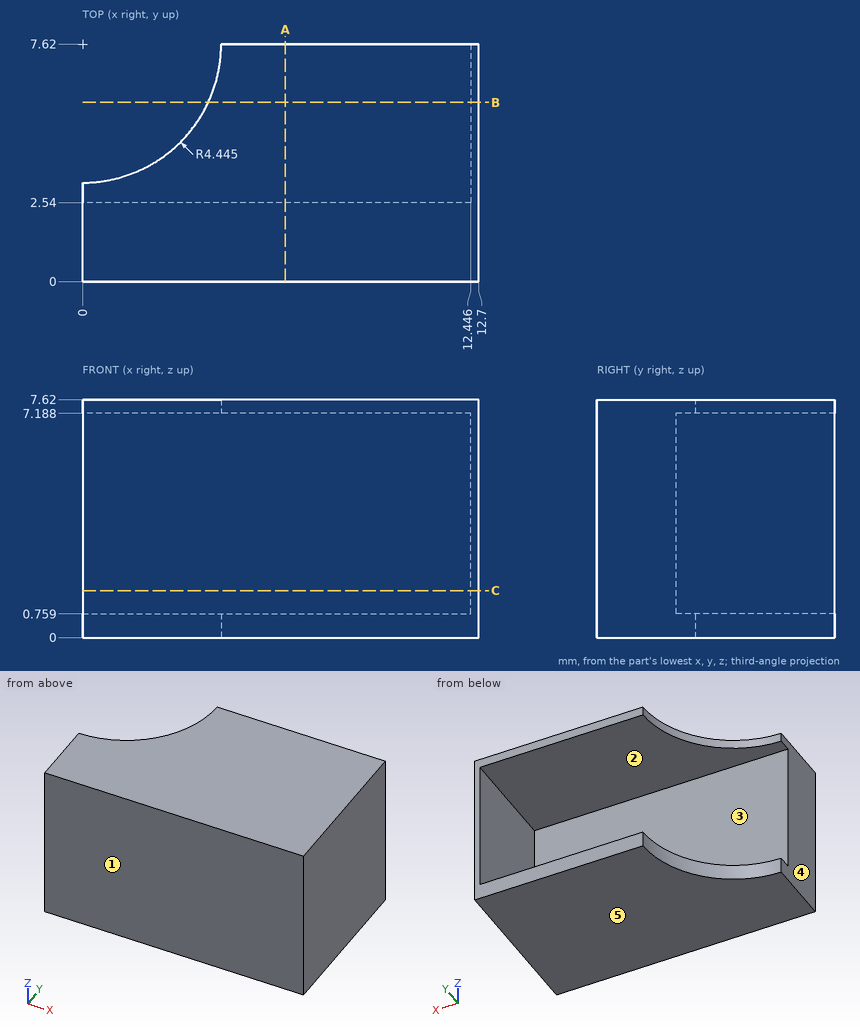
For this review, use the dimensioned drawing (mm, ordinates from the lowest corner) and the shaded views. A direction names the side the tool comes from. Coordinates: 2 decimals unless noted, no trailing zeros. Order: outer loops, then holes, each group sorted by start corner. A loop starts at its lowest first (then second) coordinate and runs counter-clockwise, first axis right, second up. Notation, with made-up numbers: (-26.5, 50.25) -> (3.5, 50.25) arc R19 cw to (3.5, 59.25) -> close; hole circle Ø4 at (-10, -35.75). An arc over 180 degrees is marked (long way). One line per item, written item: value. Start each with the question number.
Q1. Take a section at A-A, the plane x = 6.5. State the section outline as (y, z) points, then the cut area to 3 significant figures.
Q2. Take a section at C-C, the plane z = 1.5. State the section outline as (x, y) points.
Q3. For probe 1 along Z at (x, y) = (7, 4); probe 2 along X at (y, z) = (5, 2); probe 3 along Y at (x, z) = (11.25, 2.5), list the stretches that pass through material, from the lowest coordinate up.
Q4. Take a section at B-B, the plane y = 5.75. State the section outline as (x, z) points.
Q5. Insertion check: pin 1 Ø1.5 at (x, z) = (6, 3) entering from +Y. The pin has a flat end and moves straight along its axis. Give the tip position at first contact, or say it passes through.
Q6. Tool access review of the marked faces 1 and 2: name each direction out of +Z, -Z, +X, -X, +Y, -Y from which nothing blocks a thin tool from reaching the whole face with its end or side.
Q7. Mouldability with a two-part tool opening along Z and no side actions: class the marked faces 3, 4 and 5 as pulls with the +Z half, pulls with the -Z half, needs draft (parallel to the pull), parting line crosses it, or undercut.
Values follow:
1. outline: (0, 0) -> (7.62, 0) -> (7.62, 0.76) -> (2.54, 0.76) -> (2.54, 7.19) -> (7.62, 7.19) -> (7.62, 7.62) -> (0, 7.62) -> close
1. area: 25.4 mm2
2. outline: (0, 0) -> (12.7, 0) -> (12.7, 7.62) -> (12.45, 7.62) -> (12.45, 2.54) -> (0, 2.54) -> close
3. probe 1: z = 0 to 0.76, 7.19 to 7.62
3. probe 2: x = 12.45 to 12.7
3. probe 3: y = 0 to 2.54
4. outline: (4.03, 0) -> (12.7, 0) -> (12.7, 7.62) -> (4.03, 7.62) -> (4.03, 7.19) -> (12.45, 7.19) -> (12.45, 0.76) -> (4.03, 0.76) -> close
5. pin 1: stops at y = 2.54
6. face 1: +Z, -Z, +X, -X, -Y
6. face 2: -X, +Y
7. face 3: undercut
7. face 4: needs draft
7. face 5: pulls with the -Z half
